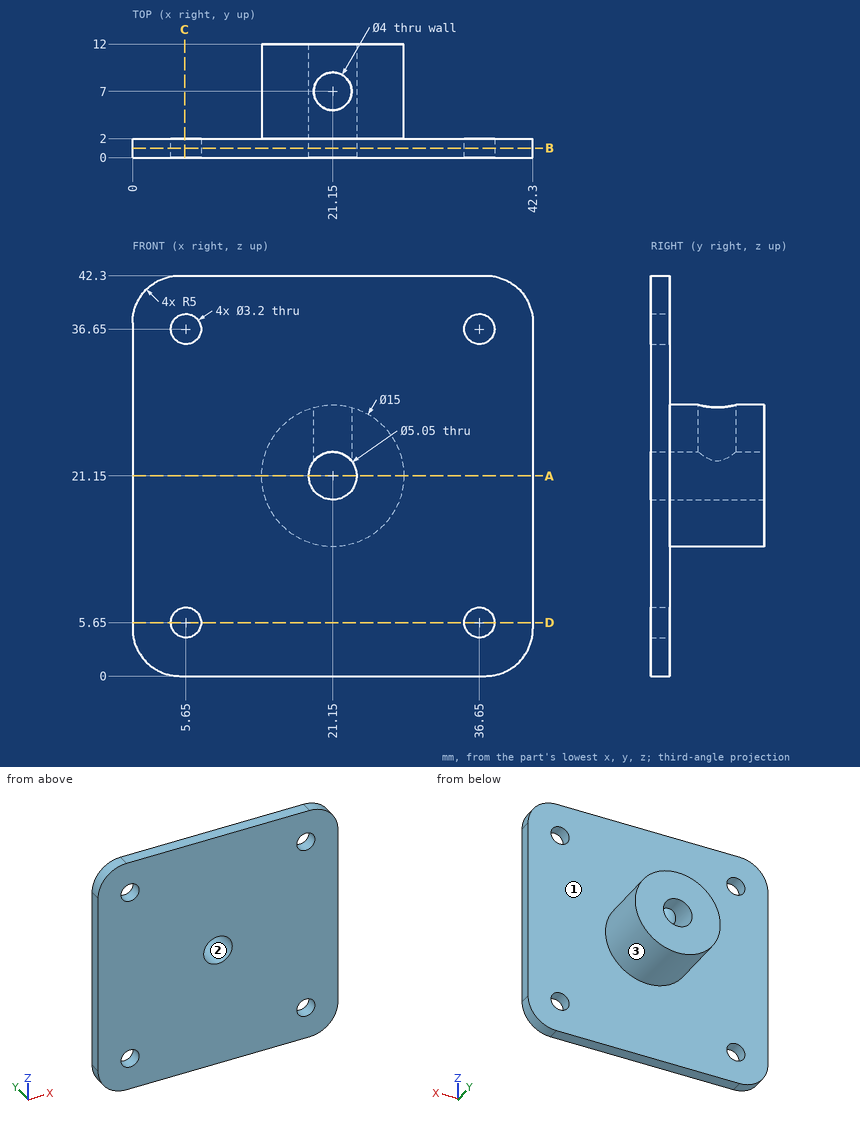
Design review of the part shown in the three views and the two pictorial views. Dimensions are in mm from the part's minimum x, y and z. Round coordinates to 2 decimals unless told otherwise and drop trailing zeros. Order: outer loops, then holes, each group sorted by start corner. A loop starts at its lowest first (then second) coordinate and runs counter-clockwise, first axis right, second up. Notation, with made-up numbers: (21.5, -5) -> (52.5, -5) arc R9 cw to (52.5, 1) -> close; hole circle Ø8 at (45.25, 14). An arc over 180 degrees is marked (long way). Write item = value, one per line. Start each with the question number.
1) Take a section at C-C on x = 5.5. State the section outline as (y, z) points.
2) The part is to be moulded in two halves that separate along X. For the marked faces 1, 2 and 3, say which applies: +X half, -X half, draft (parallel to the pull), parting line (faces both ways), or undercut.
3) Take a section at B-B on y = 1. State the section outline as (x, z) points (3 decimals).
4) Take a section at D-D on z = 5.65. State the section outline as (x, y) points.
5) Insertion check: pin 1 (6.5 mm diameter, centred on x = 21.15, y = 7, fed in from +Z); pin 2 (1 mm diameter, centred on x = 4.5, z = 32.5, fed in from +Y); pin 3 (1.5 mm diameter, centred on y = 7, z = 20, fed in from -X). Each pin has a flat end and moves straight along its axis. Give the tip position at first contact, or say it passes through.
6) To check wall thickness, follow line 1 (X direction, y = 1.05, z = 5.65); line 2 (Z direction, x = 21.15, y = 9.75) (3 decimals). State the ranges of each line that lie inside material, in increasing order. Write a range as from..to.
7) Take a section at A-A on z = 21.15. State the section outline as (x, y) points (3 decimals).
Verdict:
q1.outline = (0, 0) -> (2, 0) -> (2, 4.06) -> (0, 4.06) -> close; (0, 7.24) -> (2, 7.24) -> (2, 35.06) -> (0, 35.06) -> close; (0, 38.24) -> (2, 38.24) -> (2, 42.3) -> (0, 42.3) -> close
q2.face_1 = draft
q2.face_2 = undercut
q2.face_3 = parting line
q3.outline = (0, 5) arc R5 ccw to (5, 0) -> (37.3, 0) arc R5 ccw to (42.3, 5) -> (42.3, 37.3) arc R5 ccw to (37.3, 42.3) -> (5, 42.3) arc R5 ccw to (0, 37.3) -> close; hole circle Ø3.2 at (5.65, 5.65); hole circle Ø3.2 at (5.65, 36.65); hole circle Ø5.05 at (21.15, 21.15); hole circle Ø3.2 at (36.65, 5.65); hole circle Ø3.2 at (36.65, 36.65)
q4.outline = (0, 0) -> (4.05, 0) -> (4.05, 2) -> (0, 2) -> close; (7.25, 0) -> (35.05, 0) -> (35.05, 2) -> (7.25, 2) -> close; (38.25, 0) -> (42.3, 0) -> (42.3, 2) -> (38.25, 2) -> close
q5.pin_1 = 28.65
q5.pin_2 = 2
q5.pin_3 = 13.66
q6.line_1 = 0..4.05, 7.25..35.05, 38.25..42.3
q6.line_2 = 13.65..18.625, 23.675..28.65
q7.outline = (0, 0) -> (18.625, 0) -> (18.625, 12) -> (13.65, 12) -> (13.65, 2) -> (0, 2) -> close; (23.675, 0) -> (42.3, 0) -> (42.3, 2) -> (28.65, 2) -> (28.65, 12) -> (23.675, 12) -> close
